from build123d import *

# Parameters (mm, degrees)
M5_CLEARANCE_HOLE1_D = 5.5
FILLET1_R            = 0.2
CHAMFER1_SIZE        = 0.5
SKETCH7_R            = 14
CUT_EXTRUDE2_DEPTH   = 57.903426962
CHAMFER2_SIZE        = 0.5


with BuildPart() as part:
    # Sketch1 → Revolve1 (revolve)
    with BuildSketch(Plane.XY, mode=Mode.PRIVATE) as revolve1_sk:
        Polygon((14, -3), (14, 8), (12, 8), (12, 11), (19, 11), (19, 0), (39, 0), (39, -3), align=None)
    revolve(revolve1_sk.sketch.rotate(Axis((0, 17.954019247, 0), (0, -1, 0)), 90), axis=Axis((0, 17.954019247, 0), (0, -1, 0)))

    # M5 Clearance Hole1 (through all)
    with Locations(Plane(origin=(0, 0, 0), x_dir=(1, 0, 0), z_dir=(0, 1, 0))):
        with Locations((0, 29), (29, 0), (0, -29), (-29, 0)):
            Hole(M5_CLEARANCE_HOLE1_D / 2)

    # Fillet1
    fillet1_edges = [part.edges().sort_by_distance(p)[0] for p in [
        (0, 0, -19),
        (0, 8, -14),
    ]]
    fillet(fillet1_edges, radius=FILLET1_R)

    # Chamfer1
    chamfer1_edges = [part.edges().sort_by_distance(p)[0] for p in [
        (0, 8, -12),
        (0, 11, -12),
        (0, 11, -19),
        (0, 0, -39),
        (0, -3, -39),
        (0, -3, -14),
    ]]
    chamfer(chamfer1_edges, length=CHAMFER1_SIZE)

    # Sketch7 → Cut-Extrude2 (cut, through all)
    with BuildSketch(Plane.XZ.offset(3)):
        with Locations(Location((0, 0, 0), (0, 0, 90))):
            Circle(SKETCH7_R)
    extrude(amount=-CUT_EXTRUDE2_DEPTH, mode=Mode.SUBTRACT)

    # Chamfer2
    chamfer2_edges = [part.edges().sort_by_distance(p)[0] for p in [
        (0, 11, -14),
    ]]
    chamfer(chamfer2_edges, length=CHAMFER2_SIZE)


solid = part.part
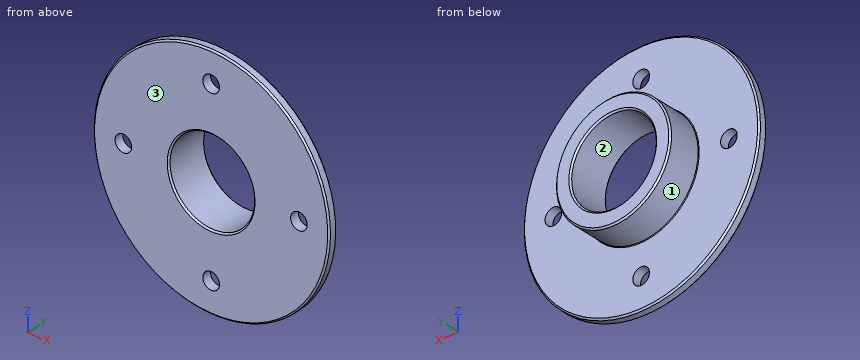
For this review, take the finished solid that the model builds, in its own axes (mm). Face numbers are marked on the shaded views. Give positions to 0.01 mm unless a question says otherwise; leave off trailing zeros. Order: outer loops, then holes, each group sorted by start corner. A loop starts at its lowest first (then second) coordinate and runs counter-clockwise, first axis right, second up. Notation, with made-up numbers: (45, 10) - (72, 10) arc R14 cw to (72, 26) - close; hole circle Ø8 at (13.25, 59). An arc over 180 degrees is marked (long way). Answer as a JSON object with one key per item and string values. Group by question number.
Item 1: Draft analysis for pull direction X (two halves, no side actions). For the marked faces 1, 2 and 3, state which applies: pulls with the +X half, pulls with the -X half, needs draft (parallel to the pull), parting line crosses it, or undercut.
Item 2: Take a section at A-A on z = 0. Give the number of separate pieces and of enclosed holes in the cut face, and give its area (3 significant figures).
Item 3: Clearance check with flat-ended pins moving along their axes: pin 1 Ø4 at (y, z) = (1, -13) entering from +X; pin 2 Ø6.5 at (x, z) = (29, 0) entering from +Y; pin 3 Ø8 at (y, z) = (5, -18) entering from +X. State where each tip first meets the part, or that it passes through.
Item 4: Take a section at C-C on y = 9.5. Give the boundary of the cut face in (x, z).
Item 5: Wall thickness on line 1 along Y through (x, z) = (-15, -22.5); line 2 along X through (y, z) = (6.5, 0); line 3 along Z through (x, y) = (29, -2.05): over which ranges is each line inside the solid? List them lowest first.
Reported:
{
 "1": {"face 1": "parting line crosses it", "face 2": "undercut", "face 3": "needs draft"},
 "2": {"separate pieces": "4", "enclosed holes": "0", "area": "226 mm^2"},
 "3": {"pin 1": "x = 37.21", "pin 2": "y = 0", "pin 3": "x = 12.85"},
 "4": {"outline": "circle Ø38 at (0, 0); hole circle Ø28 at (0, 0)"},
 "5": {"line 1": "-3 to 0", "line 2": "-19 to -14, 14 to 19", "line 3": "-26.08 to -2.75, 2.75 to 26.08"}
}
